Could you check a few things on this model? Use its own coordinates, in mm. A direction names the side the tool comes from. Give positions to 0.01 mm unless a question says otherwise; leave off trailing zeros. Order: outer loops, then holes, each group sorted by start corner. A loop starts at its lowest first (then second) coordinate and runs counter-clockwise, first axis right, second up. Notation, with made-up numbers: (57, 47) - (100, 47) arc R18 ccw to (100, 76) - close; hole circle Ø9 at (74, 34). An arc over 180 degrees is marked (long way). One line per question, with ' | ' between items. Start each with the question number.
1. Imagine slicing it at A-A (x = -339). Please give me the cut outline in (y, z), and give its area (3 significant figures).
2. Which directions (+Z, -Z, +X, -X, +Y, -Y) give clear straight access to the entire face, cutting with the end or side of a thin tool? Please do faces 1 (the flat face through (-9, -609.6, 488)), 2 (the flat face through (-8, 607.06, 490)).
3. Imagine slicing it at B-B (z = 880.5). Please give me the cut outline in (x, y), and give its area (3 significant figures).
4. If we mould it in two halves opening along Y, with no side actions, what happens to faces 3 (the flat face through (-607.06, -8, 490)), 4 (the flat face through (609.6, -9, 488)), 5 (the flat face through (-9, 609.6, 488))? For each: released by +Y, released by -Y, zero draft, split by the parting line, or undercut.
5. I need wall thicknesses on probe 1 along Y at (x, z) = (223.5, 921.5); probe 2 along Z at (x, y) = (-276, 167.5). Which ranges of each line are inside material? Lowest first, please. Write a range as from..to.
6. For P1, Ø5, axis at x = 24.5, y = -3, coming from the -Z side; P2, Ø6, axis at x = -334.5, y = -40, coming from the +Z side, each with a flat end and sliding along its axis, tell me the tip position at first contact or that it passes through.
```python
from build123d import *

# Parameters (mm, degrees)
F0_W     = 1219.2
F0_H     = 1219.2
F1_DEPTH = 990.6
F2_T     = -2.54


# Not quite as in the source:
# - the program builds the solid bodies; features that only make, move or delete a surface that nothing else refers to are left out


with BuildPart() as f1:
    # F0 (on Top) → F1 (new body)
    with BuildSketch(Plane.XY):
        Rectangle(F0_W, F0_H)
    extrude(amount=F1_DEPTH)

    # F2
    f2_openings = [f1.faces().sort_by_distance(p)[0] for p in [
        (0, 0, 990.6),
    ]]
    offset(amount=F2_T, openings=f2_openings)


solid = f1.part
```
Results found:
1) outline: (-609.6, 0) - (609.6, 0) - (609.6, 990.6) - (607.06, 990.6) - (607.06, 2.54) - (-607.06, 2.54) - (-607.06, 990.6) - (-609.6, 990.6) - close | area: 8,120 mm2
2) face 1: +Z, -Z, +X, -X, -Y | face 2: +Z
3) outline: (-609.6, -609.6) - (609.6, -609.6) - (609.6, 609.6) - (-609.6, 609.6) - close; hole (-607.06, -607.06) - (607.06, -607.06) - (607.06, 607.06) - (-607.06, 607.06) - close | area: 12,400 mm2
4) face 3: undercut | face 4: zero draft | face 5: released by +Y
5) probe 1: y = -609.6..-607.06, 607.06..609.6 | probe 2: z = 0..2.54
6) P1: stops at z = 0 | P2: stops at z = 2.54
